from build123d import *

# Parameters (mm, degrees)
F3_DEPTH = 5.081
F5_DEPTH = 2.54
F6_R     = 2.286
F7_DEPTH = 2.541


with BuildPart() as f1:
    # F0 (on Front) → F1 (revolve)
    with BuildSketch(Plane.XZ):
        with BuildLine():
            Line((0, 5.08), (-31.75, 5.08))
            ThreePointArc((-31.75, 5.08), (-30.779806, 2.54), (-31.75, 0))
            Line((-31.75, 0), (0, 0))
            Line((0, 0), (0, 5.08))
        make_face()
    revolve(axis=Axis((0, 0, 2.54), (0, 0, -1)))

    # F2 (on face) → F3 (cut, through all)
    with BuildSketch(Plane.XY.offset(5.08)):
        with BuildLine():
            Line((-5.08, -5.08), (-26.181721, -5.08))
            ThreePointArc((-26.181721, -5.08), (-18.858538, -18.858538), (-5.08, -26.181721))
            Line((-5.08, -26.181721), (-5.08, -5.08))
        make_face()
        with BuildLine():
            ThreePointArc((-5.08, 26.181721), (-18.858538, 18.858538), (-26.181721, 5.08))
            Line((-26.181721, 5.08), (-5.08, 5.08))
            Line((-5.08, 5.08), (-5.08, 26.181721))
        make_face()
        with BuildLine():
            Line((5.08, -5.08), (5.08, -26.181721))
            ThreePointArc((5.08, -26.181721), (18.858538, -18.858538), (26.181721, -5.08))
            Line((26.181721, -5.08), (5.08, -5.08))
        make_face()
        with BuildLine():
            Line((5.08, 5.08), (26.181721, 5.08))
            ThreePointArc((26.181721, 5.08), (18.858538, 18.858538), (5.08, 26.181721))
            Line((5.08, 26.181721), (5.08, 5.08))
        make_face()
    extrude(amount=-F3_DEPTH, mode=Mode.SUBTRACT)

    # F4 (on face) → F5 (cut)
    with BuildSketch(Plane.XY.offset(5.08)):
        Polygon((-6.2357, 3.600183), (-6.2357, -3.600183), (0, -7.200366), (6.2357, -3.600183), (6.2357, 3.600183), (0, 7.200366), align=None)
    extrude(amount=-F5_DEPTH, mode=Mode.SUBTRACT)

    # F6 (on face) → F7 (cut, through all)
    with BuildSketch(Plane.XY.offset(2.54)):
        Circle(F6_R)
    extrude(amount=-F7_DEPTH, mode=Mode.SUBTRACT)


solid = f1.part
Input: part model. Units: mm. Frame: model coordinates. A direction names the side the tool comes from. Give positions to 0.01 mm unless a question says otherwise; leave off trailing zeros. Loops run counter-clockwise (first coordinate to the right, second up) from the corner with the lowest first, then second, coordinate; pieces in that order, holes last. Notation, with made-up numbers: M 76.5,41 L 84.5,41 A26 cw 84.5,70 Z; hole C -11,32 d1. An arc over 180 degrees is marked long. Use CSV: the item, a comma, the result in double quotes.
(1) Section C-C, the plane x = -12.5. Count the separate pieces of the cut face and the enclosed holes in it, plus the area to 3 significant figures.
Outcome:
separate pieces,"3"
enclosed holes,"0"
area,"101 mm²"
(2) Pin query (flat end, axial travel): P1, Ø2, axis at y = -1.5, z = 3.5, coming from the +X side; P2, Ø2, axis at y = 0.5, z = 4, coming from the -X side; P3, Ø2, axis at x = -21, z = 4, coming from the +Y side; P4, Ø2.5, axis at x = 0, y = 0, coming from the +Z side. Return the tip coordinate at first contact, or that it passes through.
Outcome:
P1,"stops at x = 31.29"
P2,"stops at x = -31.68"
P3,"stops at y = 24.04"
P4,"passes through"
(3) Section A-A, the plane y = 0. Return loops of the section in (x, z).
Outcome:
outline,"M -31.75,0 L -2.29,0 L -2.29,2.54 L -6.24,2.54 L -6.24,5.08 L -31.75,5.08 A3.81 cw Z; M 2.29,0 L 31.75,0 A3.81 cw 31.75,5.08 L 6.24,5.08 L 6.24,2.54 L 2.29,2.54 Z"
(4) Set-up query: faces 1 (the face through (7, 0, 5.08)), 2 (the face through (5.08, -15, 3)), 3 (the face through (3.07, -5.43, 3.83)). Return all of +Z, -Z, +X, -X, +Y, -Y with unobstructed straight access to the full face (end or side cutting, diameter ignored); none if empty.
Outcome:
face 1,"+Z, +X, -X, +Y, -Y"
face 2,"+Z, -Z"
face 3,"+Z"
(5) Section B-B, the plane z = 3.85. Return loops of the section in (x, y), plus the area to 3 significant figures.
Outcome:
outline,"C 0,0 d62.02; hole M -26.18,-5.08 A26.67 ccw -5.08,-26.18 L -5.08,-5.08 Z; hole M -26.18,5.08 L -5.08,5.08 L -5.08,26.18 A26.67 ccw Z; hole M -6.24,-3.6 L 0,-7.2 L 6.24,-3.6 L 6.24,3.6 L 0,7.2 L -6.24,3.6 Z; hole M 5.08,-26.18 A26.67 ccw 26.18,-5.08 L 5.08,-5.08 Z; hole M 5.08,5.08 L 26.18,5.08 A26.67 ccw 5.08,26.18 Z"
area,"1,630 mm²"
(6) Material intervals for L1, parallel to X at y = 15, z = 4; L2, parallel to Y at x = 21.5, z = 3.6; L3, parallel to Y at x = -18.5, z = 4.1, sorted ascending. Write a range as [from, to].
Outcome:
L1,"x = [-27.21, -22.05], [-5.08, 5.08], [22.05, 27.21]"
L2,"y = [-22.24, -15.78], [-5.08, 5.08], [15.78, 22.24]"
L3,"y = [-25.02, -19.21], [-5.08, 5.08], [19.21, 25.02]"
(7) Pull-direction query (X, two-part tool) for faces 4 (the face through (0, -7, 0)), 5 (the face through (3.161, 5.375, 3.828)); classes: pulls with the +X half, pulls with the -X half, needs draft (parallel to the pull), parting line crosses it, or undercut.
Outcome:
face 4,"needs draft"
face 5,"undercut"
